Work out the finished part from the listing and answer in its coordinate system (mm). A direction names the side the tool comes from. Coordinates: 2 decimals unless noted, no trailing zeros. Loops run counter-clockwise (first coordinate to the right, second up) from the corner with the lowest first, then second, coordinate; pieces in that order, holes last. Notation, with made-up numbers: (-23, -12.75) -> (11, -12.75) arc R12 cw to (11, -3.75) -> close; hole circle Ø2 at (85, 44.5). An arc over 180 degrees is marked (long way). Use a Markdown table: item, result. Add a question column.
```python
from build123d import *

# Parameters (mm, degrees)
CROQUIS1_R              = 36.29
SALIENTE_EXTRUIR1_DEPTH = 1.25
CROQUIS2_W              = 29.94
CROQUIS2_H              = 54.01
CROQUIS2_W_2            = 27.94
CROQUIS2_H_2            = 52.01
SALIENTE_EXTRUIR2_DEPTH = 5
CROQUIS3_R              = 2.60731142
CROQUIS3_R_2            = 1.60731142
CROQUIS3_R_3            = 2.6
CROQUIS3_R_4            = 1.6
CROQUIS3_R_5            = 2.600000001
CROQUIS3_R_6            = 1.600000001
SALIENTE_EXTRUIR3_DEPTH = 5.59
CROQUIS3_3_R            = 1.60731142
CROQUIS3_3_R_2          = 1.6
CROQUIS3_3_R_3          = 1.600000001
CORTAR_EXTRUIR1_DEPTH   = 8.5


with BuildPart() as part:
    # Croquis1 → Saliente-Extruir1 (new body, symmetric)
    with BuildSketch(Plane(origin=(0, 0, 0), x_dir=(1, 0, 0), z_dir=(0, 1, 0))):
        Circle(CROQUIS1_R)
    extrude(amount=SALIENTE_EXTRUIR1_DEPTH, both=True)

    # Croquis2 → Saliente-Extruir2 (add)
    with BuildSketch(Plane.XZ.offset(1.25)):
        Rectangle(CROQUIS2_W, CROQUIS2_H)
        Rectangle(CROQUIS2_W_2, CROQUIS2_H_2, mode=Mode.SUBTRACT)
    extrude(amount=SALIENTE_EXTRUIR2_DEPTH)

    # Croquis3 → Saliente-Extruir3 (add)
    with BuildSketch(Plane(origin=(0, 1.25, 0), x_dir=(1, 0, 0), z_dir=(0, 1, 0))):
        with Locations((-14, 30)):
            Circle(CROQUIS3_R)
        with Locations((-14, 30)):
            Circle(CROQUIS3_R_2, mode=Mode.SUBTRACT)
        with Locations((14, 30)):
            Circle(CROQUIS3_R_3)
        with Locations((14, 30)):
            Circle(CROQUIS3_R_4, mode=Mode.SUBTRACT)
        with Locations((-14.000000001, -30)):
            Circle(CROQUIS3_R_5)
        with Locations((-14.000000001, -30)):
            Circle(CROQUIS3_R_6, mode=Mode.SUBTRACT)
        with Locations((13.999999999, -30)):
            Circle(CROQUIS3_R_5)
        with Locations((13.999999999, -30)):
            Circle(CROQUIS3_R_6, mode=Mode.SUBTRACT)
    extrude(amount=SALIENTE_EXTRUIR3_DEPTH)

    # Croquis3_3 → Cortar-Extruir1 (cut, through all)
    with BuildSketch(Plane(origin=(0, 1.25, 0), x_dir=(1, 0, 0), z_dir=(0, 1, 0))):
        with Locations((-14, 30)):
            Circle(CROQUIS3_3_R)
        with Locations((14, 30)):
            Circle(CROQUIS3_3_R_2)
        with Locations((-14.000000001, -30)):
            Circle(CROQUIS3_3_R_3)
        with Locations((13.999999999, -30)):
            Circle(CROQUIS3_3_R_3)
    extrude(amount=-CORTAR_EXTRUIR1_DEPTH, mode=Mode.SUBTRACT)


solid = part.part
```
Item 1: For a pull along Z with two mould halves and no side action, classify faces 1 (the face through (-14.5, -6.25, 8.1)), 2 (the face through (0, -4, 27.005)), 3 (the face through (-14.56, 4.01, 32.54)) as +Z half, -Z half, draft (parallel to the pull), parting line (faces both ways), or undercut.
Item 2: Section D-D (z = 0) is taken. Determine the outline of the cut face in (x, y), then the cut area to 3 significant figures.
Item 3: Section C-C (y = -5) is taken. Determine the outline of the cut face in (x, z) (3 decimals), then the cut area to 3 significant figures.
Item 4: Find the intervals of material crossed by probe 1 along Z at (x, y) = (14, 3.9); probe 2 along Z at (x, y) = (-13.5, -3) (3 decimals); probe 3 along X at (y, z) = (-0.1, 30), in increasing order.
Item 5: Section B-B (x = 0) is taken. Determine the outline of the cut face in (y, z) (3 decimals), then the cut area to 3 significant figures.
Item 6: For faces 4 (the face through (14.97, -4, 0)), 5 (the face through (13.44, 4.01, 32.54)), 6 (the face through (0, -4, 26.005)), 7 (the face through (-14.97, -4, 0)), determine the directions among +Z, -Z, +X, -X, +Y, -Y from which every point of the face is accessible in a straight line to the end or side of a thin tool.
Item 7: Given pin 1 (1.5 mm diameter, centred on x = 9.5, y = 0, fed in from +Z); pin 2 (4 mm diameter, centred on x = 2, y = -3, fed in from +Z); pin 3 (1.5 mm diameter, centred on x = 7.5, y = -4.5, fed in from +Z) (3 decimals), each flat-ended and moving along its own axis, determine where each tip first touches the part or whether it passes through.
Item 8: Section A-A (z = -30) is taken. Determine the outline of the cut face in (x, y).
Output:
| question | item | result |
|---|---|---|
| 1 | face 1 | draft |
| 1 | face 2 | +Z half |
| 1 | face 3 | undercut |
| 2 | outline | (-36.29, -1.25) -> (-14.97, -1.25) -> (-14.97, -6.25) -> (-13.97, -6.25) -> (-13.97, -1.25) -> (13.97, -1.25) -> (13.97, -6.25) -> (14.97, -6.25) -> (14.97, -1.25) -> (36.29, -1.25) -> (36.29, 1.25) -> (-36.29, 1.25) -> close |
| 2 | area | 191 mm2 |
| 3 | outline | (-14.97, -27.005) -> (14.97, -27.005) -> (14.97, 27.005) -> (-14.97, 27.005) -> close; hole (-13.97, -26.005) -> (13.97, -26.005) -> (13.97, 26.005) -> (-13.97, 26.005) -> close |
| 3 | area | 164 mm2 |
| 4 | probe 1 | z = -32.6 to -31.6, -28.4 to -27.4, 27.4 to 28.4, 31.6 to 32.6 |
| 4 | probe 2 | z = -27.005 to -26.005, 26.005 to 27.005 |
| 4 | probe 3 | x = -20.42 to -15.6, -12.4 to 12.4, 15.6 to 20.42 |
| 5 | outline | (-6.25, -27.005) -> (-1.25, -27.005) -> (-1.25, -36.29) -> (1.25, -36.29) -> (1.25, 36.29) -> (-1.25, 36.29) -> (-1.25, 27.005) -> (-6.25, 27.005) -> (-6.25, 26.005) -> (-1.25, 26.005) -> (-1.25, -26.005) -> (-6.25, -26.005) -> close |
| 5 | area | 191 mm2 |
| 6 | face 4 | +Z, -Z, +X, -Y |
| 6 | face 5 | +Y |
| 6 | face 6 | -Y |
| 6 | face 7 | +Z, -Z, -X, -Y |
| 7 | pin 1 | stops at z = 35.22 |
| 7 | pin 2 | stops at z = 36.28 |
| 7 | pin 3 | stops at z = 27.005 |
| 8 | outline | (-20.42, -1.25) -> (-15.61, -1.25) -> (-15.61, 6.84) -> (-16.61, 6.84) -> (-16.61, 1.25) -> (-20.42, 1.25) -> close; (-12.39, -1.25) -> (12.4, -1.25) -> (12.4, 6.84) -> (11.4, 6.84) -> (11.4, 1.25) -> (-11.39, 1.25) -> (-11.39, 6.84) -> (-12.39, 6.84) -> close; (15.6, -1.25) -> (20.42, -1.25) -> (20.42, 1.25) -> (16.6, 1.25) -> (16.6, 6.84) -> (15.6, 6.84) -> close |
